```python
from build123d import *

# Parameters (mm, degrees)
SKETCH1_R           = 2.125
BOSS_EXTRUDE1_DEPTH = 3
BOSS_EXTRUDE2_DEPTH = 3


with BuildPart() as part:
    # Sketch1 → Boss-Extrude1 (new body)
    with BuildSketch(Plane(origin=(0, 0, 0), x_dir=(1, 0, 0), z_dir=(0, 1, 0))):
        with BuildLine():
            Line((-30, 4), (30, 4))
            ThreePointArc((30, 4), (34, 0), (30, -4))
            Line((30, -4), (-30, -4))
            ThreePointArc((-30, -4), (-34, 0), (-30, 4))
        make_face()
        with Locations(Location((30, 0, 0), (0, 0, 270))):
            Circle(SKETCH1_R, mode=Mode.SUBTRACT)
        with Locations(Location((5, 0, 0), (0, 0, 270))):
            Circle(SKETCH1_R, mode=Mode.SUBTRACT)
    extrude(amount=BOSS_EXTRUDE1_DEPTH)

    # Sketch3 → Boss-Extrude2 (add)
    with BuildSketch(Plane.XZ):
        Polygon((-30, 4), (-20, 6.679491924), (-20, 4), align=None)
    extrude(amount=-BOSS_EXTRUDE2_DEPTH)


solid = part.part
```
Model file for the job. Use its own axes, mm. A direction names the side the tool comes from. Give positions to 0.01 mm unless a question says otherwise; leave off trailing zeros. Loops run counter-clockwise (first coordinate to the right, second up) from the corner with the lowest first, then second, coordinate; pieces in that order, holes last. Notation, with made-up numbers: (86.25, 57.5) - (91.25, 57.5) arc R17 ccw to (91.25, 64.5) - close; hole circle Ø2 at (85.5, 81). An arc over 180 degrees is marked (long way). One line per item, written item: value. Start each with the question number.
1. Pin check, flat tips, straight feed: pin 1 (0.8 mm diameter, centred on y = 1, z = 6, fed in from +X); pin 2 (4 mm diameter, centred on x = -2.5, z = 4.5, fed in from -Y); pin 3 (4 mm diameter, centred on x = 5, z = 0, fed in from -Y). Stop position of each tip, or through.
2. Which spindle directions (+Z, -Z, +X, -X, +Y, -Y) get a long thin tool onto all of the face, cutting with end or side? Do faces 5 (the flat face through (5, 1, 4)), 6 (the flat face through (0, 0, 0)). Say none if no direction does.
3. Slice it at C-C (y = 1.15). Give the number of separate pieces and of enclosed holes in the cut face, plus the area to 3 significant figures.
4. Probe L1, parallel to X at y = 1.05, z = 0 (3 decimals); L2, parallel to X at y = 1.65, z = 1.25; L3, parallel to Z at x = 17, y = 2.05. List the from-to ranges inside material, lowest first. Write a range as from..to.
5. Slice it at A-A (z = 0). List the corners of the cut face in (x, y) (3 decimals).
6. Slice it at D-D (x = -27). List the corners of the cut face in (y, z), plus the area to 3 significant figures.
7. Pull direction X, two halves, no side cores. Call faces 1 (the cylindrical face through (34, 1, 0)), 2 (the flat face through (0, 1, -4)), 3 (the cylindrical face through (2.926, 1.479, -0.461)), 4 (the cylindrical face through (-34, 1, 0)): pulls with the +X half, pulls with the -X half, needs draft (parallel to the pull), parting line crosses it, or undercut.
8. Slice it at B-B (x = 5). List the corners of the cut face in (y, z) (3 decimals).
Solution:
1. pin 1: stops at x = -20
1. pin 2: stops at y = 0
1. pin 3: passes through
2. face 5: +Z, +X, +Y, -Y
2. face 6: +Z, -Z, +X, -X, -Y
3. separate pieces: 1
3. enclosed holes: 2
3. area: 515 mm^2
4. L1: x = -34..2.875, 7.125..27.875, 32.125..34
4. L2: x = -33.8..3.28, 6.72..28.28, 31.72..33.8
4. L3: z = -4..4
5. outline: (-34, 0) - (2.875, 0) - (2.875, 3) - (-34, 3) - close; (7.125, 0) - (27.875, 0) - (27.875, 3) - (7.125, 3) - close; (32.125, 0) - (34, 0) - (34, 3) - (32.125, 3) - close
6. outline: (0, -4) - (3, -4) - (3, 4.8) - (0, 4.8) - close
6. area: 26.4 mm^2
7. face 1: pulls with the +X half
7. face 2: needs draft
7. face 3: undercut
7. face 4: pulls with the -X half
8. outline: (0, -4) - (3, -4) - (3, -2.125) - (0, -2.125) - close; (0, 2.125) - (3, 2.125) - (3, 4) - (0, 4) - close
